Here's how the part is built. I have some questions about the finished solid (model axes, mm). Round coordinates to 2 decimals unless told otherwise and drop trailing zeros. Order: outer loops, then holes, each group sorted by start corner. A loop starts at its lowest first (then second) coordinate and runs counter-clockwise, first axis right, second up.
```python
from build123d import *

# Parameters (mm, degrees)
F0_W     = 28.057197
F0_H     = 82.694904
F1_DEPTH = 25.4
F4_D     = 5.1054
F5_D     = 5.1054


with BuildPart() as f1:
    # F0 (on Top) → F1 (new body)
    with BuildSketch(Plane.XY):
        with Locations((-19.532638, -10.070052)):
            Rectangle(F0_W, F0_H)
    extrude(amount=F1_DEPTH)

    # F4 (through all)
    with Locations(Plane.YZ.offset(-5.50404)):
        with Locations((19.304432, 13.261723), (-6.095568, 13.261723), (-31.495568, 13.261723)):
            Hole(F4_D / 2)

    # F5 (through all)
    with Locations(Plane.XY.offset(25.4)):
        with Locations((-22.04302, 21.531211), (-22.04302, -3.868789), (-22.04302, -29.268789)):
            Hole(F5_D / 2)


solid = f1.part
```
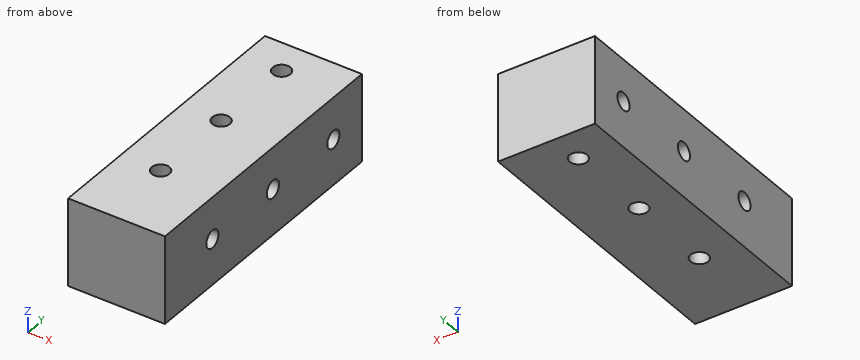
1. If we section it at C-C, the plane z = 1.5: Write out the boundary of the cut face in (x, y).
Evaluation:
outline: (-33.56, -51.42) - (-5.5, -51.42) - (-5.5, 31.28) - (-33.56, 31.28) - close; hole circle Ø5.11 at (-22.04, -29.27); hole circle Ø5.11 at (-22.04, -3.87); hole circle Ø5.11 at (-22.04, 21.53)
2. If we section it at B-B, the plane x = -21.75: Write out the boundary of the cut face in (y, z), and give its area (3 significant figures).
Evaluation:
outline: (-51.42, 0) - (-31.8, 0) - (-31.8, 10.73) arc R2.55 cw to (-31.8, 15.8) - (-31.8, 25.4) - (-51.42, 25.4) - close; (-26.73, 0) - (-6.4, 0) - (-6.4, 10.73) arc R2.55 cw to (-6.4, 15.8) - (-6.4, 25.4) - (-26.73, 25.4) - close; (-1.33, 0) - (19, 0) - (19, 10.73) arc R2.55 cw to (19, 15.8) - (19, 25.4) - (-1.33, 25.4) - close; (24.07, 0) - (31.28, 0) - (31.28, 25.4) - (24.07, 25.4) - close
area: 1,690 mm2
3. If we section it at A-A, the plane y = 18: Write out the boundary of the cut face in (x, z).
Evaluation:
outline: (-33.56, 0) - (-5.5, 0) - (-5.5, 11.07) - (-33.56, 11.07) - close; (-33.56, 15.46) - (-5.5, 15.46) - (-5.5, 25.4) - (-33.56, 25.4) - close
4. I need wall thicknesses on probe 1 along Z at (x, y) = (-9, -6); probe 2 along Y at (x, z) = (-23.75, 22.5); probe 3 along Y at (x, z) = (-20.25, 24.25). Which ranges of each line are inside material? Lowest first, please.
Evaluation:
probe 1: z = 0 to 10.71, 15.81 to 25.4
probe 2: y = -51.42 to -31.17, -27.37 to -5.77, -1.97 to 19.63, 23.43 to 31.28
probe 3: y = -51.42 to -31.09, -27.45 to -5.69, -2.05 to 19.71, 23.35 to 31.28
5. If we section it at D-D, the plane x = -29: Write out the boundary of the cut face in (y, z).
Evaluation:
outline: (-51.42, 0) - (31.28, 0) - (31.28, 25.4) - (-51.42, 25.4) - close; hole circle Ø5.11 at (-31.5, 13.26); hole circle Ø5.11 at (-6.1, 13.26); hole circle Ø5.11 at (19.3, 13.26)
